Autodesk Inventor part; units mm, degrees
ref_plane "YZ Plane" through (0, 0, 0) normal (1, 0, 0) x (0, 1, 0)
ref_plane "XZ Plane" through (0, 0, 0) normal (0, 1, 0) x (-1, 0, 0)
ref_plane "XY Plane" through (0, 0, 0) normal (0, 0, 1) x (1, 0, 0)
sketch "Sketch1" plane through (0, 0, 0) normal (0, 1, 0) x (-1, 0, 0)
  circle A0 centre (0, 0) radius 6.4585
  dimension "d0" = 12.917
extrude "Extrusion1" add sketch "Sketch1" along normal blind 11
sketch "Sketch2" plane through (0, 11, 0) normal (0, 1, 0) x (1, 0, 0)
  circle A0 centre (0, 0) radius 6.4585
  circle A1 centre (0, 0) radius 6
  dimension "d3" = 12
extrude "Extrusion2" add sketch "Sketch2" along normal blind 5 contours A1
sketch "Sketch3" plane through (0, 0, 0) normal (1, 0, 0) x (0, 1, 0)
  line L0 (16, -6) -> (16, 6)
  line L1 (16, -4.8) -> (22.2, -4.8)
  line L2 (22.2, 0) -> (16, 0)
  arc A0 (22.2, -4.8) -> (27, 0) centre (22.2, 0) ccw
  line L3 (0, 6.4585) -> (0, -6.4585)
  line L4 (22.2, 0) -> (27, 0)
  line L5 (16, 0) -> (27, 0)
  point P0 (0, 0)
  dimension "d7" = 4.8
  dimension "d13" = 22.2
revolve "Revolution1" add sketch "Sketch3" angle 360 about axis through (0, 16, 0) along (0, 1, 0)
sketch "Sketch4" plane through (0, 16, 0) normal (0, 1, 0) x (1, 0, 0)
  circle A0 centre (0, 0) radius 4.8
  circle A1 centre (0, 0) radius 6
  line L0 (2.5, -11.2443) -> (-2.5, -11.2443)
  line L1 (-2.5, 11.2443) -> (2.5, 11.2443)
  line L2 (2.5, -11.2443) -> (-2.5, 11.2443) construction
  line L3 (-2.5, -11.2443) -> (2.5, 11.2443) construction
  circle A2 centre (0, 0) radius 4.8
  line L4 (2.5, 11.2443) -> (2.5, 5.4544)
  line L5 (3.1579, 3.6149) -> (3.1579, -3.6149)
  line L6 (-3.1579, -3.6149) -> (-3.1579, 3.6149)
  dimension "d9" = 5
extrude "Extrusion3" cut sketch "Sketch4" along normal blind 13.25 contours A0 L5 | L6 A0
hole "Hole1" at (3.1579, 22.2, 0) direction (-1, 0, 0) diameter 6.1 depth 8 tip angle 118
thread "Thread1"
thread "Thread2"
sketch "Sketch5" plane through (0, 0, 0) normal (0, -1, 0) x (1, 0, 0)
  circle A0 centre (0, 0) radius 6.4585
  circle A1 centre (0, 0) radius 6
  dimension "d27" = 12
hole "Hole2" at (0, 0, 0) direction (0, 1, 0) diameter 10.917 depth 10
ref_plane "Work Plane1" through (-0.8421, 22.2, 0) normal (0, -1, 0) x (1, 0, 0)
sketch "Sketch6" plane through (-0.8421, 22.2, 0) normal (0, -1, 0) x (1, 0, 0)
  circle A0 centre (0.8421, 0) radius 3.3
  line L0 (4.1421, 0) -> (-2.4579, 0)
  line L1 (4, 3.05) -> (4, -3.05)
  line L2 (-8.1998, 0) -> (9.884, 0)
  dimension "d36" = 6.6
revolve "Revolution2" cut sketch "Sketch6" angle 360 about axis through (-0.8421, 22.2, 0) along (1, 0, 0) picked at (4.0262, 0.5339) picked at (-0.2745, 0.2585) contours L0 L1 A0 | L1 L0 A0
properties part number "500-106" material "Stainless Steel"
Input: part model. Units: mm. Frame: model coordinates. A direction names the side the tool comes from. Give positions to 0.01 mm unless a question says otherwise; leave off trailing zeros. Write each loop counter-clockwise with the first axis right and the second up, starting at its lowest first coordinate (ties: lowest second). Pieces come first, ordered by that corner, then holes. Notation, with made-up numbers: (-20.75, 60) - (5.25, 60) arc R14 cw to (5.25, 83) - close; hole circle Ø9 at (52.5, 65.25). An arc over 180 degrees is marked (long way). Write item = value, one per line. Start each with the question number.
1) Cut plane B-B (x = 0). Return loops of the section in (y, z), and give its area (3 significant figures).
2) Material intervals for L1, parallel to Z at x = 0, y = 6.25; L2, parallel to Z at x = -4.75, y = 7.25; L3, parallel to X at y = 5.5, z = -3.5, sorted ascending. Write a range as [from, to].
3) Pin query (flat end, axial travel): pin 1 (2 mm diameter, centred on x = 2, y = 6.5, fed in from -Z); pin 2 (3.5 mm diameter, centred on y = 22.2, z = 0, fed in from -X); pin 3 (2 mm diameter, centred on x = 1, y = 14.5, fed in from +Z); pin 4 (3.5 mm diameter, centred on x = -1.5, z = -2.5, fed in from -Y). Return the tip coordinate at first contact, or that it passes through.
4) Draft query along X for faces 5 (the face through (-3.158, 19, 0)), 6 (the face through (-6, 13, 0)), 7 (the face through (0, 10, 0)), 8 (the face through (4, 16, 0)). Return one class per face: pulls with the +X half, pulls with the -X half, needs draft (parallel to the pull), parting line crosses it, or undercut.
5) Cut plane C-C (y = 23.75). Return loops of the section in (x, z), and give its area (3 significant figures).
6) Reachability of faces 1 (the face through (3.158, 19, 0)), 2 (the face through (0, 19.1, -4.8)), 3 (the face through (5.33, 5.07, 1.18)), 4 (the face through (0, 19.1, 4.8)) from +Z, -Z, +X, -X, +Y, -Y: full face, straight path, thin tool, end or side. Return the list, or none.
7) Cut plane D-D (x = -4). Return loops of the section in (y, z).
8) Cut plane A-A (z = 0). Return loops of the section in (x, y), and give its area (3 significant figures).
Answers follow:
q1.outline = (0, -6.46) - (11, -6.46) - (11, -6) - (16, -6) - (16, -4.8) - (22.2, -4.8) arc R4.8 ccw to (22.2, 4.8) - (16, 4.8) - (16, 6) - (11, 6) - (11, 6.46) - (0, 6.46) - (0, 5.46) - (10, 5.46) - (10, -5.46) - (0, -5.46) - close; hole circle Ø6.6 at (22.2, 0)
q1.area = 154 mm^2
q2.L1 = [-6.46, -5.46], [5.46, 6.46]
q2.L2 = [-4.38, -2.69], [2.69, 4.38]
q2.L3 = [-5.43, -4.19], [4.19, 5.43]
q3.pin_1 = -6.38
q3.pin_2 = through
q3.pin_3 = 6
q3.pin_4 = 10
q4.face_5 = pulls with the -X half
q4.face_6 = parting line crosses it
q4.face_7 = undercut
q4.face_8 = needs draft
q5.outline = (-3.16, -3.27) arc R4.54 ccw to (3.16, -3.27) - (3.16, -2.63) - (1.26, -2.63) arc R2.91 cw to (-1.26, -2.63) - (-3.16, -2.63) - close; (-3.16, 2.63) - (-1.26, 2.63) arc R2.91 cw to (1.26, 2.63) - (3.16, 2.63) - (3.16, 3.27) arc R4.54 ccw to (-3.16, 3.27) - close
q5.area = 18.2 mm^2
q6.face_1 = +Z, -Z, +X, +Y
q6.face_2 = -Z, +Y
q6.face_3 = -Y
q6.face_4 = +Z, +Y
q7.outline = (0, -5.07) - (11, -5.07) - (11, -4.47) - (16, -4.47) - (16, 4.47) - (11, 4.47) - (11, 5.07) - (0, 5.07) - (0, 3.71) - (10, 3.71) - (10, -3.71) - (0, -3.71) - close
q8.outline = (-6.46, 0) - (-5.46, 0) - (-5.46, 10) - (5.46, 10) - (5.46, 0) - (6.46, 0) - (6.46, 11) - (6, 11) - (6, 16) - (3.16, 16) - (3.16, 19.15) - (1.26, 19.15) arc R3.3 cw to (-1.26, 19.15) - (-3.16, 19.15) - (-3.16, 16) - (-6, 16) - (-6, 11) - (-6.46, 11) - close; (-3.16, 25.25) - (-1.26, 25.25) arc R3.3 cw to (1.26, 25.25) - (3.16, 25.25) - (3.16, 25.81) arc R4.8 ccw to (-3.16, 25.81) - close
q8.area = 121 mm^2
